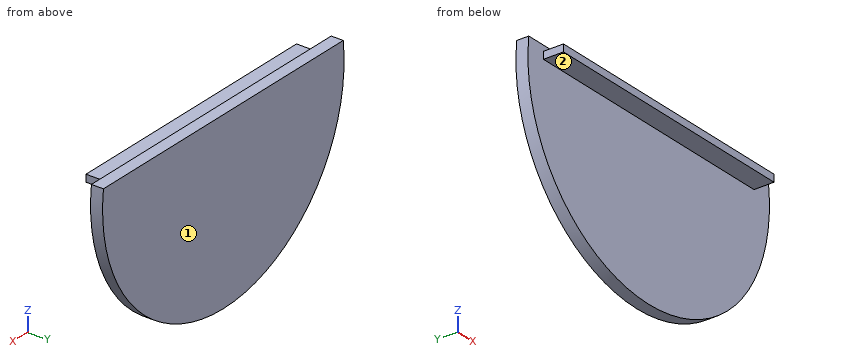
from build123d import *

# Parameters (mm, degrees)
SKETCH1_R           = 39
BOSS_EXTRUDE1_DEPTH = 3
SKETCH3_W           = 110.988465814
SKETCH3_H           = 40.72920708
CUT_EXTRUDE1_DEPTH  = 3
SKETCH4_W           = 68
SKETCH4_H           = 1.8
BOSS_EXTRUDE2_DEPTH = 5
SKETCH4_2_W         = 68
SKETCH4_2_H         = 1.8
BOSS_EXTRUDE3_DEPTH = 5


with BuildPart() as part:
    # Sketch1 → Boss-Extrude1 (new body)
    with BuildSketch(Plane(origin=(0, 0, 0), x_dir=(1, 0, 0), z_dir=(0, 1, 0))):
        Circle(SKETCH1_R)
    extrude(amount=BOSS_EXTRUDE1_DEPTH)

    # Sketch3 → Cut-Extrude1 (cut)
    with BuildSketch(Plane(origin=(0, 3, 0), x_dir=(1, 0, 0), z_dir=(0, 1, 0))):
        with Locations((0.606471885, -24.96460354)):
            Rectangle(SKETCH3_W, SKETCH3_H)
    extrude(amount=-CUT_EXTRUDE1_DEPTH, mode=Mode.SUBTRACT)

    # Sketch4 → Boss-Extrude2 (add)
    with BuildSketch(Plane.XZ):
        with Locations((0, 2.3)):
            Rectangle(SKETCH4_W, SKETCH4_H)
    extrude(amount=BOSS_EXTRUDE2_DEPTH)

    # Sketch4<2> → Boss-Extrude3 (add)
    with BuildSketch(Plane.XZ):
        with Locations((0, 2.3)):
            Rectangle(SKETCH4_2_W, SKETCH4_2_H)
    extrude(amount=BOSS_EXTRUDE3_DEPTH)


solid = part.part
The model under review builds one solid part; all positions refer to its coordinate system, in mm. Face numbers are marked on the shaded views. A direction names the side the tool comes from. Give positions to 0.01 mm unless a question says otherwise; leave off trailing zeros. Order: outer loops, then holes, each group sorted by start corner. A loop starts at its lowest first (then second) coordinate and runs counter-clockwise, first axis right, second up. Notation, with made-up numbers: (20, 45) -> (59, 45) arc R18 cw to (59, 80) -> close; hole circle Ø6 at (50, 16.25). An arc over 180 degrees is marked (long way). Write item = value, one per line. Start each with the question number.
(1) Take a section at B-B (z = 0). Write out the cut boundary in (x, y).
(2) Take a section at A-A (x = 0). Write out the cut boundary in (y, z).
(3) Take a section at C-C (y = -1.75). Write out the cut boundary in (x, z), plus the area to 3 significant figures.
(4) Tool access review of the marked faces 1 and 2: name each direction out of +Z, -Z, +X, -X, +Y, -Y from which nothing blocks a thin tool from reaching the whole face with its end or side.
(5) For L1, parallel to Y at x = -6, z = -14.5; L2, parallel to Z at x = -18, y = -2.5; L3, parallel to X at y = 1.5, z = -17, list the stretches that pass through material, from the lowest coordinate up. Write a range as from..to.
(6) Take a section at D-D (x = -30). Write out the cut boundary in (y, z), plus the area to 3 significant figures.
(7) For pin 1 Ø2 at (y, z) = (-3.5, 2) entering from +X; pin 2 Ø2 at (y, z) = (-2.5, -23.5) entering from -X; pin 3 Ø0.5 at (y, z) = (-2.5, 2) entering from -X; pin 4 Ø4 at (x, y) = (-10.5, -2.5) entering from -Z, all flat-tipped, find the tip position at first contact; note any pin that passes through.
Returned:
q1.outline = (-39, 0) -> (39, 0) -> (39, 3) -> (-39, 3) -> close
q2.outline = (-5, 1.4) -> (0, 1.4) -> (0, -39) -> (3, -39) -> (3, 4.6) -> (0, 4.6) -> (0, 3.2) -> (-5, 3.2) -> close
q3.outline = (-34, 1.4) -> (34, 1.4) -> (34, 3.2) -> (-34, 3.2) -> close
q3.area = 122 mm²
q4.face_1 = +Z, -Z, +X, -X, +Y
q4.face_2 = -Z, +X, -X, -Y
q5.L1 = 0..3
q5.L2 = 1.4..3.2
q5.L3 = -35.1..35.1
q6.outline = (-5, 1.4) -> (0, 1.4) -> (0, -24.92) -> (3, -24.92) -> (3, 4.6) -> (0, 4.6) -> (0, 3.2) -> (-5, 3.2) -> close
q6.area = 97.6 mm²
q7.pin_1 = 34
q7.pin_2 = through
q7.pin_3 = -34
q7.pin_4 = 1.4
